For this review, take the finished solid that the model builds, in its own axes (mm). A direction names the side the tool comes from. Round coordinates to 2 decimals unless told otherwise and drop trailing zeros. Loops run counter-clockwise (first coordinate to the right, second up) from the corner with the lowest first, then second, coordinate; pieces in that order, holes last.
1) Mouldability with a two-part tool opening along Z and no side actions: class faces 4 (the flat face through (-41, 41, -31.75)), 5 (the cylindrical face through (26.803, 40.697, -17.02)), 6 (the flat face through (25, 82.55, 0)) as pulls with the +Z half, pulls with the -Z half, needs draft (parallel to the pull), parting line crosses it, or undercut.
2) Take a section at A-A (y = 19.05). State the section outline as (x, z) points (3 decimals).
3) Wall thickness on L1, parallel to Y at x = -57.15, z = -23.5 (3 decimals); L2, parallel to X at y = 19, z = -23; L3, parallel to X at y = 19, z = -27: over which ranges is each line inside the solid? List them lowest first.
4) Insertion check: pin 1 (8 mm diameter, centred on x = -2.5, y = 9, fed in from +Z); pin 2 (10 mm diameter, centred on x = -6.5, y = 60, fed in from -Z). Each pin has a flat end and moves straight along its axis. Give the tip position at first contact, or say it passes through.
5) Take a section at B-B (z = -19.05). State the section outline as (x, y) points (3 decimals).
6) Tool access review of faces 1 (the flat face through (76.2, 59, -23)), 2 (the flat face through (85.86, 12.52, -44.27)), 3 (the cylindrical face through (85.86, 57.14, -16.98)): name each direction out of +Z, -Z, +X, -X, +Y, -Y from which nothing blocks a thin tool from reaching the whole face with its end or side.
7) Take a section at C-C (x = -57.15). State the section outline as (y, z) points (3 decimals).
8) Take a section at D-D (y = 7). State the section outline as (x, z) points (3 decimals), then the cut area to 3 significant figures.
```python
from build123d import *

# Parameters (mm, degrees)
SKETCH1_R           = 15.875
BOSS_EXTRUDE1_DEPTH = 82.55
SKETCH2_R           = 15.875
CUT_EXTRUDE1_DEPTH  = 41.402
SKETCH3_R           = 9.525
CUT_EXTRUDE2_DEPTH  = 41.402
CHAMFER1_SIZE       = 25.4
CHAMFER2_SIZE       = 25.4


with BuildPart() as part:
    # Sketch1 → Boss-Extrude1 (new body)
    with BuildSketch(Plane(origin=(0, 0, 0), x_dir=(1, 0, 0), z_dir=(0, 1, 0))):
        with BuildLine():
            Line((0, 31.75), (-82.55, 31.75))
            Line((-82.55, 31.75), (-82.55, 12.7))
            Line((-82.55, 12.7), (-29.099355663, 12.7))
            ThreePointArc((-29.099355663, 12.7), (-26.563955842, -17.390191201), (0, -31.75))
            Line((0, -31.75), (95.25, -31.75))
            Line((95.25, -31.75), (95.25, 57.15))
            Line((95.25, 57.15), (76.2, 57.15))
            Line((76.2, 57.15), (76.2, -12.7))
            Line((76.2, -12.7), (29.099355663, -12.7))
            ThreePointArc((29.099355663, -12.7), (26.563955842, 17.390191201), (0, 31.75))
        make_face()
        Circle(SKETCH1_R, mode=Mode.SUBTRACT)
    extrude(amount=BOSS_EXTRUDE1_DEPTH)

    # Sketch2 → Cut-Extrude1 (cut)
    with BuildSketch(Plane(origin=(95.25, 0, 0), x_dir=(0, 0, -1), z_dir=(1, 0, 0))):
        with Locations((19.05, 41.402)):
            Circle(SKETCH2_R)
    extrude(amount=-CUT_EXTRUDE1_DEPTH, mode=Mode.SUBTRACT)

    # Sketch3 → Cut-Extrude2 (cut)
    with BuildSketch(Plane(origin=(0, 0, -31.75), x_dir=(-1, 0, 0), z_dir=(0, 0, -1))):
        with Locations((57.15, 63.5)):
            Circle(SKETCH3_R)
        with Locations((57.15, 19.05)):
            Circle(SKETCH3_R)
    extrude(amount=-CUT_EXTRUDE2_DEPTH, mode=Mode.SUBTRACT)

    # Chamfer1
    chamfer1_edges = [part.edges().sort_by_distance(p)[0] for p in [
        (85.725, 82.55, -57.15),
    ]]
    chamfer(chamfer1_edges, length=CHAMFER1_SIZE)

    # Chamfer2
    chamfer2_edges = [part.edges().sort_by_distance(p)[0] for p in [
        (85.725, 0, -57.15),
    ]]
    chamfer(chamfer2_edges, length=CHAMFER2_SIZE)


solid = part.part
```
Response:
1. face 4: pulls with the -Z half
1. face 5: undercut
1. face 6: needs draft
2. outline: (-82.55, -31.75) - (-66.675, -31.75) - (-66.675, -12.7) - (-82.55, -12.7) - close; (-47.625, -31.75) - (0, -31.75) arc R31.75 ccw to (29.099, 12.7) - (76.2, 12.7) - (76.2, -50.8) - (95.25, -50.8) - (95.25, 31.75) - (0, 31.75) arc R31.75 ccw to (-29.099, -12.7) - (-47.625, -12.7) - close; hole circle Ø31.75 at (0, 0)
3. L1: y = 0 to 9.525, 28.575 to 53.975, 73.025 to 82.55
3. L2: x = -82.55 to -66.67, -47.63 to 21.89, 76.2 to 95.25
3. L3: x = -82.55 to -66.67, -47.63 to 16.71, 76.2 to 95.25
4. pin 1: stops at z = 31.75
4. pin 2: stops at z = -31.75
5. outline: (-82.55, 0) - (25.4, 0) - (25.4, 82.55) - (-82.55, 82.55) - close; (76.2, 0) - (95.25, 0) - (95.25, 25.527) - (76.2, 25.527) - close; (76.2, 57.277) - (95.25, 57.277) - (95.25, 82.55) - (76.2, 82.55) - close; hole circle Ø19.05 at (-57.15, 19.05); hole circle Ø19.05 at (-57.15, 63.5)
6. face 1: -Z, +Y, -Y
6. face 2: -Z, +X, -X, -Y
6. face 3: +X
7. outline: (0, -31.75) - (9.525, -31.75) - (9.525, -12.7) - (0, -12.7) - close; (28.575, -31.75) - (53.975, -31.75) - (53.975, -12.7) - (28.575, -12.7) - close; (73.025, -31.75) - (82.55, -31.75) - (82.55, -12.7) - (73.025, -12.7) - close
8. outline: (-82.55, -31.75) - (0, -31.75) arc R31.75 ccw to (29.099, 12.7) - (76.2, 12.7) - (76.2, -38.75) - (95.25, -38.75) - (95.25, 31.75) - (0, 31.75) arc R31.75 ccw to (-29.099, -12.7) - (-82.55, -12.7) - close; hole circle Ø31.75 at (0, 0)
8. area: 5,940 mm2
